```python
from build123d import *

# Parameters (mm, degrees)
SKETCH_1_R             = 62
SKETCH_1_R_2           = 60
EXTRUDE_1_DEPTH        = 3
EXTRUDE_START          = 6
SKETCH_2_R             = 48
EXTRUDE_2_DEPTH        = 6
FILLET_1_R             = 5
CHAMFER_1_SIZE         = 0.5
CHAMFER_2_SIZE         = 0.5
SKETCH_6_R             = 2.2
CUT_EXTRUDE_1_DEPTH    = 6
SKETCH_7_W             = 65
SKETCH_7_H             = 13.477482046
EXTRUDE_3_DEPTH        = 3
SKETCH_11_R            = 1.65
CUT_EXTRUDE_2_DEPTH    = 3
CHAMFER_3_SIZE         = 1
CHAMFER_4_SIZE         = 1
FILLET_2_R             = 3
CHAMFER_5_3_ANGLE      = 291.929687
SKETCH_12_R            = 4
CUT_EXTRUDE_3_DEPTH    = 3
CUT_EXTRUDE_4_DEPTH    = 2
CHAMFER_6_SIZE         = 1
HOLE_WIZARD_M3_1_D     = 2.5
HOLE_WIZARD_M3_1_DEPTH = 7.5
HOLE_WIZARD_M3_1_TIP   = 0.751075774


with BuildPart() as part:
    # 草图1 → 凸台-拉伸1 (new body)
    with BuildSketch(Plane.XY):
        Circle(SKETCH_1_R)
        Circle(SKETCH_1_R_2, mode=Mode.SUBTRACT)
    extrude(amount=-EXTRUDE_1_DEPTH)

    # 草图2 → 凸台-拉伸2 (add)
    with BuildSketch(Plane.XY.offset(EXTRUDE_START)):
        with BuildLine():
            Line((-32.5, 63), (32.5, 63))
            Line((32.5, 63), (32.5, 52.79914772))
            ThreePointArc((32.5, 52.79914772), (0, -62), (-32.5, 52.79914772))
            Line((-32.5, 52.79914772), (-32.5, 63))
        make_face()
        Circle(SKETCH_2_R, mode=Mode.SUBTRACT)
    extrude(amount=-EXTRUDE_2_DEPTH)

    # 圆角1
    # the kernel refuses this fillet: 5 mm, written as the material it adds along each edge
    with BuildSketch(Plane(origin=(32.5, 52.79914772, 6), x_dir=(0.8403342947446245, -0.5420685132675156, 0), z_dir=(0, 0, -1))) as fillet_1_piece_1:
        with BuildLine():
            CenterArc((2.72541822, -4.998883971), FILLET_1_R, 91.210593649, 55.964843523)
            Line((-1.476253254, -2.288541405), (0, 0))
            ThreePointArc((0, 0), (1.309890927, -0.013838756), (2.619781855, 0))
        make_face()
    extrude(amount=6)
    with BuildSketch(Plane(origin=(-32.5, 52.79914772, 6), x_dir=(-0.840334294744627, -0.5420685132675117, 0), z_dir=(0, 0, -1))) as fillet_1_piece_2:
        with BuildLine():
            CenterArc((2.72541822, 4.998883971), FILLET_1_R, 212.824562828, 55.964843523)
            Line((-1.476253254, 2.288541405), (0, 0))
            ThreePointArc((0, 0), (1.309890927, 0.013838756), (2.619781855, 0))
        make_face()
    extrude(amount=6)

    # 倒角1
    chamfer_1_edges = [part.edges().sort_by_distance(p)[0] for p in [
        (-48, 0, 0),
        (-48, 0, 6),
        (-60, 0, -3),
    ]]
    chamfer(chamfer_1_edges, length=CHAMFER_1_SIZE)

    # 倒角2
    # the kernel refuses this chamfer: 0.5 mm, written as the material it takes off along each edge
    with BuildSketch(Plane(origin=(-32.5, 55.522517954, 0), x_dir=(0, 0, 1), z_dir=(0, 1, 0)), Plane(origin=(32.5, 64.285841494, 0), x_dir=(0, 0, 1), z_dir=(0, -1, 0))) as chamfer_2_piece_1:
        Polygon((CHAMFER_2_SIZE, 0), (0, CHAMFER_2_SIZE), (0, 0), align=None)
    extrude(amount=8.76332354, mode=Mode.SUBTRACT)
    with BuildSketch(Plane(origin=(37.5, 55.522517954, 0), x_dir=(-0.15613015555825177, -0.9877364904291813, 0), z_dir=(0.9877364904291813, -0.15613015555825177, 0))) as chamfer_2_piece_2_section:
        Polygon((5, -CHAMFER_2_SIZE), (5 + CHAMFER_2_SIZE, 0), (5, 0), align=None)
    chamfer_2_piece_2 = revolve(axis=Axis((37.5, 55.522517954, 0), (0, 0, -1)), revolution_arc=81.017652556, mode=Mode.PRIVATE)
    chamfer_2_piece_2 = chamfer_2_piece_2 - Plane(origin=(0, 0, 0), x_dir=(1, 0, 0), z_dir=(0, 0, 1)) * Cylinder(62, 22, mode=Mode.PRIVATE)
    add(chamfer_2_piece_2, mode=Mode.SUBTRACT)
    with BuildSketch(Plane(origin=(-37.5, 55.522517954, 0), x_dir=(1, 0, 0), z_dir=(0, 1, 0))) as chamfer_2_piece_3_section:
        Polygon((5, -CHAMFER_2_SIZE), (5 + CHAMFER_2_SIZE, 0), (5, 0), align=None)
    chamfer_2_piece_3 = revolve(axis=Axis((-37.5, 55.522517954, 0), (0, 0, -1)), revolution_arc=81.017652556, mode=Mode.PRIVATE)
    chamfer_2_piece_3 = chamfer_2_piece_3 - Plane(origin=(0, 0, 0), x_dir=(1, 0, 0), z_dir=(0, 0, 1)) * Cylinder(62, 22, mode=Mode.PRIVATE)
    add(chamfer_2_piece_3, mode=Mode.SUBTRACT)

    # 草图6 → 切除-拉伸1 (cut)
    with BuildSketch(Plane(origin=(0, 0, 0), x_dir=(-1, 0, 0), z_dir=(0, 0, -1))):
        with Locations((-42.877900702, 31.152618372)):
            Circle(SKETCH_6_R)
        with Locations((-53, 0)):
            Circle(SKETCH_6_R)
        with Locations((-42.877900702, -31.152618371)):
            Circle(SKETCH_6_R)
        with Locations((-16.377900702, -50.405995364)):
            Circle(SKETCH_6_R)
        with Locations((16.377900702, -50.405995364)):
            Circle(SKETCH_6_R)
        with Locations((42.877900702, -31.152618371)):
            Circle(SKETCH_6_R)
        with Locations((53, 0)):
            Circle(SKETCH_6_R)
        with Locations((42.877900702, 31.152618372)):
            Circle(SKETCH_6_R)
        with Locations((16.377900702, 50.405995364)):
            Circle(SKETCH_6_R)
        with Locations((-16.377900702, 50.405995364)):
            Circle(SKETCH_6_R)
    extrude(amount=-CUT_EXTRUDE_1_DEPTH, mode=Mode.SUBTRACT)

    # 草图7 → 凸台-拉伸3 (add)
    with BuildSketch(Plane.XY.offset(6)):
        with Locations((0, 62.261258977)):
            Rectangle(SKETCH_7_W, SKETCH_7_H)
    extrude(amount=EXTRUDE_3_DEPTH)

    # 草图11 → 切除-拉伸2 (cut)
    with BuildSketch(Plane.XY.offset(9)):
        with Locations((-29.5, 66)):
            Circle(SKETCH_11_R)
        with Locations((29.5, 66)):
            Circle(SKETCH_11_R)
    extrude(amount=-CUT_EXTRUDE_2_DEPTH, mode=Mode.SUBTRACT)

    # 倒角3
    chamfer_3_edges = [part.edges().sort_by_distance(p)[0] for p in [
        (0, 63, 0),
    ]]
    chamfer(chamfer_3_edges, length=CHAMFER_3_SIZE - 0.0001)  # a hair under: the kernel refuses the full size

    # 倒角4
    chamfer_4_edges = [part.edges().sort_by_distance(p)[0] for p in [
        (0, 55.522517954, 9),
    ]]
    chamfer(chamfer_4_edges, length=CHAMFER_4_SIZE)

    # 圆角2
    fillet_2_edges = [part.edges().sort_by_distance(p)[0] for p in [
        (-32.5, 69, 7.5),
        (32.5, 69, 7.5),
    ]]
    fillet(fillet_2_edges, radius=FILLET_2_R)

    # 倒角5: read off the stored shape, not the designer's step
    # 倒角5 outline → 倒角5 (revolve, cut)
    with BuildSketch(Plane(origin=(37.5, 55.522517954, 0), x_dir=(1, 0, 0), z_dir=(0, -1, 0))):
        Polygon((4.999998721, 9), (4.999998721, 4.999998721), (9, 9), align=None)
    revolve(axis=Axis((37.5, 55.522517954, 0), (0, 0, 1)), mode=Mode.SUBTRACT)

    # Chamfer 5 2 outline → Chamfer 5 2 (revolve, cut)
    with BuildSketch(Plane(origin=(-37.5, 55.522517954, 0), x_dir=(1, 0, 0), z_dir=(0, -1, 0))):
        Polygon((4.99999762, 9), (4.99999762, 4.99999762), (9, 9), align=None)
    revolve(axis=Axis((-37.5, 55.522517954, 0), (0, 0, 1)), mode=Mode.SUBTRACT)

    # Chamfer 5 3 outline → Chamfer 5 3 (revolve, cut)
    with BuildSketch(Plane(origin=(0, 0, 0), x_dir=(-0.5597014925373135, 0.8286942978273132, 0), z_dir=(0.8286942978273132, 0.5597014925373135, 0))):
        Polygon((62, 6), (61, 6), (62, 5), align=None)
    revolve(axis=Axis((0, 0, 0), (0, 0, 1)), revolution_arc=CHAMFER_5_3_ANGLE, mode=Mode.SUBTRACT)

    # 草图12 → 切除-拉伸3 (cut)
    with BuildSketch(Plane.XY.offset(6)):
        with Locations((-16.377900702, 50.405995364)):
            Circle(SKETCH_12_R)
        with Locations((16.377900702, 50.405995364)):
            Circle(SKETCH_12_R)
        with Locations((42.877900702, 31.152618372)):
            Circle(SKETCH_12_R)
        with Locations((53, 0)):
            Circle(SKETCH_12_R)
        with Locations((42.877900702, -31.152618371)):
            Circle(SKETCH_12_R)
        with Locations((16.377900702, -50.405995364)):
            Circle(SKETCH_12_R)
        with Locations((-16.377900702, -50.405995364)):
            Circle(SKETCH_12_R)
        with Locations((-42.877900702, -31.152618371)):
            Circle(SKETCH_12_R)
        with Locations((-53, 0)):
            Circle(SKETCH_12_R)
        with Locations((-42.877900702, 31.152618372)):
            Circle(SKETCH_12_R)
    extrude(amount=-CUT_EXTRUDE_3_DEPTH, mode=Mode.SUBTRACT)

    # 草图14 → 切除-拉伸4 (cut)
    with BuildSketch(Plane(origin=(0, 63, 0), x_dir=(1, 0, 0), z_dir=(0, 1, 0))):
        with BuildLine():
            ThreePointArc((-4.030108666, 3.809429698), (-11.733833556, 7.447967709), (-11.5, -1.068584287))
            ThreePointArc((-11.5, -1.068584287), (0, -4.15), (11.5, -1.068584287))
            ThreePointArc((11.5, -1.068584287), (11.733833556, 7.447967709), (4.030108666, 3.809429698))
            ThreePointArc((4.030108666, 3.809429698), (0, 5.85), (-4.030108666, 3.809429698))
        make_face()
    extrude(amount=-CUT_EXTRUDE_4_DEPTH, mode=Mode.SUBTRACT)

    # 倒角6
    # the kernel refuses this chamfer: 1 mm, written as the material it takes off along each edge
    with BuildSketch(Plane(origin=(18.80558547, 61, -3), x_dir=(0, -1, 0), z_dir=(-1, 0, 0))) as chamfer_6_piece_1:
        Polygon((CHAMFER_6_SIZE, 0), (0, CHAMFER_6_SIZE), (0, 0), align=None)
    extrude(amount=37.61117094, mode=Mode.SUBTRACT)
    with BuildSketch(Plane(origin=(-9, 63, -3.261542732), x_dir=(-0.874686173337968, 0, 0.48468969266055384), z_dir=(-0.48468969266055384, 0, -0.874686173337968))) as chamfer_6_piece_2:
        Polygon((5, -CHAMFER_6_SIZE), (5 + CHAMFER_6_SIZE, 0), (5, 0), align=None)
    revolve(axis=Axis((-9, 63, -3.261542732), (0, 1, 0)), revolution_arc=31.007856081, mode=Mode.SUBTRACT)
    with BuildSketch(Plane(origin=(9, 63, -3.261542732), x_dir=(0.49999999999998873, 0, 0.8660254037844451), z_dir=(-0.8660254037844451, 0, 0.49999999999998873))) as chamfer_6_piece_3:
        Polygon((5, -CHAMFER_6_SIZE), (5 + CHAMFER_6_SIZE, 0), (5, 0), align=None)
    revolve(axis=Axis((9, 63, -3.261542732), (0, 1, 0)), revolution_arc=31.007856081, mode=Mode.SUBTRACT)
    with BuildSketch(Plane(origin=(0, 63, -18.85), x_dir=(-0.500000000000001, 0, 0.8660254037844382), z_dir=(-0.8660254037844382, 0, -0.500000000000001))) as chamfer_6_piece_4:
        Polygon((23, -CHAMFER_6_SIZE), (23 + CHAMFER_6_SIZE, 0), (23, 0), align=None)
    revolve(axis=Axis((0, 63, -18.85), (0, 1, 0)), revolution_arc=60, mode=Mode.SUBTRACT)

    # M3 螺纹孔1
    with Locations(Plane.XY.offset(9)):
        with Locations((-25, 60), (25, 60)):
            Hole(HOLE_WIZARD_M3_1_D / 2, depth=HOLE_WIZARD_M3_1_DEPTH)
            with Locations((0, 0, -(HOLE_WIZARD_M3_1_DEPTH + HOLE_WIZARD_M3_1_TIP / 2))):  # 118° drill point
                Cone(0, HOLE_WIZARD_M3_1_D / 2, HOLE_WIZARD_M3_1_TIP, mode=Mode.SUBTRACT)


solid = part.part
```
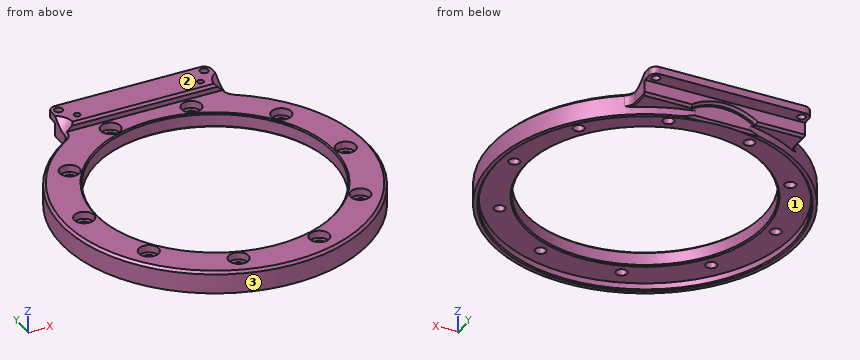
Check sheet for the modelled part. Datum: model origin and axes. Units: mm. Face numbers are marked on the shaded views. Coordinates: 2 decimals unless noted, no trailing zeros. Write item = value, one per line. Start each with the question number.
1) Cross-section at A-A (y = 0). State how many separate pieces and enclosed holes the cut face has, then the cut area to 3 significant figures.
2) Go/stop test with flat-tipped pins: P1, Ø3, axis at x = 20.5, z = -1, coming from the -Y side; P2, Ø4.5, axis at y = 61, z = 3, coming from the +X side; P3, Ø8, axis at x = -47.5, y = 10.5, coming from the +Z side; P4, Ø3.5, axis at x = -42.88, y = 31.15, coming from the +Z side. Record where each tip stops, or that it passes through.
3) Mould release check, pull along Y, two halves, no side actions. Record for the marked faces 1, 2 and 3: +Y half, -Y half, draft (parallel to the pull), parting line (faces both ways), or undercut.
4) Material ranges on L1, parallel to X at y = 59.5, z = 3; L2, parallel to X at y = 60, z = 7; L3, parallel to Y at x = -25, z = 1, recorded low to high.
Ans:
q1.separate_pieces = 4
q1.enclosed_holes = 0
q1.area = 104 mm²
q2.P1 = -59.02
q2.P2 = 32.5
q2.P3 = 6
q2.P4 = through
q3.face_1 = undercut
q3.face_2 = draft
q3.face_3 = parting line
q4.L1 = -32.5 to -26.15, -23.85 to 23.85, 26.15 to 32.5
q4.L2 = -32.12 to -26.25, -23.75 to 23.75, 26.25 to 32.12
q4.L3 = -56.74 to -40.98, 40.98 to 59.58, 60.42 to 63
